from build123d import *

# Parameters (mm, degrees)
CROQUIS1_W              = 44.6
CROQUIS1_H              = 20.647373716
SALIENTE_EXTRUIR2_DEPTH = 10.5
CROQUIS2_R              = 7.366343287
CROQUIS2_R_2            = 3.5
SALIENTE_EXTRUIR3_DEPTH = 2
SALIENTE_EXTRUIR4_START = -2
CROQUIS3_R              = 6.292932571
CROQUIS3_R_2            = 3.5
SALIENTE_EXTRUIR4_DEPTH = 2
CORTAR_EXTRUIR1_DEPTH   = 5.5
CORTAR_EXTRUIR2_DEPTH   = 5.5
CROQUIS6_W              = 8
CROQUIS6_H              = 20.647373716
SALIENTE_EXTRUIR5_DEPTH = 3
CROQUIS7_W              = 8
CROQUIS7_H              = 20.647373716
SALIENTE_EXTRUIR6_DEPTH = 3
REDONDEO1_R             = 10
REDONDEO2_R             = 2


with BuildPart() as part:
    # Croquis1 → Saliente-Extruir2 (new body)
    with BuildSketch(Plane.XY):
        Rectangle(CROQUIS1_W, CROQUIS1_H)
        Polygon((5.946707773, 0), (2.973353886, 5.15), (-2.973353886, 5.15), (-5.946707773, 0), (-2.973353886, -5.15), (2.973353886, -5.15), align=None, mode=Mode.SUBTRACT)
    extrude(amount=SALIENTE_EXTRUIR2_DEPTH)

    # Croquis2 → Saliente-Extruir3 (add)
    with BuildSketch(Plane.XY.offset(10.5)):
        Circle(CROQUIS2_R)
        Circle(CROQUIS2_R_2, mode=Mode.SUBTRACT)
    extrude(amount=-SALIENTE_EXTRUIR3_DEPTH)

    # Croquis3 → Saliente-Extruir4 (add)
    with BuildSketch(Plane(origin=(0, 0, 0), x_dir=(-1, 0, 0), z_dir=(0, 0, -1)).offset(SALIENTE_EXTRUIR4_START)):
        Circle(CROQUIS3_R)
        with Locations(Location((0, 0, 0), (0, 0, 180))):
            Circle(CROQUIS3_R_2, mode=Mode.SUBTRACT)
    extrude(amount=SALIENTE_EXTRUIR4_DEPTH)

    # Croquis4 → Cortar-Extruir1 (cut)
    with BuildSketch(Plane(origin=(22.3, 0, 0), x_dir=(0, 0, -1), z_dir=(1, 0, 0))):
        Polygon((-5.25, 6.062177826), (-10.5, 3.031088913), (-10.5, -3.031088913), (-5.25, -6.062177826), (0, -3.031088913), (0, 3.031088913), align=None)
    extrude(amount=-CORTAR_EXTRUIR1_DEPTH, mode=Mode.SUBTRACT)

    # Croquis5 → Cortar-Extruir2 (cut)
    with BuildSketch(Plane.ZY.offset(22.3)):
        Polygon((5.25, 6.062177826), (0, 3.031088913), (0, -3.031088913), (5.25, -6.062177826), (10.5, -3.031088913), (10.5, 3.031088913), align=None)
    extrude(amount=-CORTAR_EXTRUIR2_DEPTH, mode=Mode.SUBTRACT)

    # Croquis6 → Saliente-Extruir5 (add)
    with BuildSketch(Plane(origin=(0, 0, 0), x_dir=(-1, 0, 0), z_dir=(0, 0, -1))):
        with Locations((-18.3, 0)):
            Rectangle(CROQUIS6_W, CROQUIS6_H)
        with Locations((18.3, 0)):
            Rectangle(CROQUIS6_W, CROQUIS6_H)
    extrude(amount=SALIENTE_EXTRUIR5_DEPTH)

    # Croquis7 → Saliente-Extruir6 (add)
    with BuildSketch(Plane.XY.offset(10.5)):
        with Locations((-18.3, 0)):
            Rectangle(CROQUIS7_W, CROQUIS7_H)
        with Locations((18.3, 0)):
            Rectangle(CROQUIS7_W, CROQUIS7_H)
    extrude(amount=SALIENTE_EXTRUIR6_DEPTH)

    # Redondeo1
    # the kernel refuses this fillet: 10 mm, written as the material it adds along each edge
    with BuildSketch(Plane(origin=(-14.3, 10.323686858, 10.5), x_dir=(1, 0, 0), z_dir=(0, -1, 0)), Plane(origin=(14.3, 10.323686858, 0), x_dir=(-1, 0, 0), z_dir=(0, -1, 0))) as redondeo1_piece_1:
        with BuildLine():
            CenterArc((7.141428429, 10), REDONDEO1_R, 224.427004001, 45.572995999)
            Line((0, 3), (-0.142828569, 2.86))
            ThreePointArc((-0.142828569, 2.86), (-0.2, 1.5), (-0.2, 0))
            Line((-0.2, 0), (0, -0.2))
            Line((0, -0.2), (7.141428429, -0.2))
            Line((7.141428429, -0.2), (7.141428429, 0))
        make_face()
    extrude(amount=20.647373716)
    with BuildSketch(Plane(origin=(14.3, 10.323686858, 10.5), x_dir=(0, 0, 1), z_dir=(0, -1, 0)), Plane(origin=(-14.3, 10.323686858, 0), x_dir=(0, 0, -1), z_dir=(0, -1, 0))) as redondeo1_piece_2:
        with BuildLine():
            CenterArc((10, 7.141428429), REDONDEO1_R, 180, 45.572995999)
            Line((0, 7.141428429), (-0.2, 7.141428429))
            Line((-0.2, 7.141428429), (-0.2, 0))
            Line((-0.2, 0), (0, -0.2))
            ThreePointArc((0, -0.2), (1.5, -0.2), (2.86, -0.142828569))
            Line((2.86, -0.142828569), (3, 0))
        make_face()
    extrude(amount=20.647373716)

    # Redondeo2
    redondeo2_edges = [part.edges().sort_by_distance(p)[0] for p in [
        (18.3, -10.323686858, -3),
        (18.3, 10.323686858, -3),
        (-18.3, 10.323686858, -3),
        (-18.3, -10.323686858, 13.5),
        (-18.3, 10.323686858, 13.5),
        (18.3, 10.323686858, 13.5),
        (18.3, -10.323686858, 13.5),
    ]]
    fillet(redondeo2_edges, radius=REDONDEO2_R)


solid = part.part
Can you work these out from the model? Positions are in its coordinate system, mm. A direction names the side the tool comes from. Coordinates: 2 decimals unless noted, no trailing zeros. Write each loop counter-clockwise with the first axis right and the second up, starting at its lowest first coordinate (ties: lowest second). Pieces come first, ordered by that corner, then holes. Notation, with made-up numbers: (20, 68) -> (69, 68) arc R10 cw to (69, 87) -> close; hole circle Ø3 at (43.5, 81). An arc over 180 degrees is marked (long way). Answer as CSV lines item,"result".
1) Will these pins go through, and if not, where does the flat tip stop? P1, Ø3, axis at y = 3, z = 6, coming from the -X side; P2, Ø9, axis at x = 0, y = 0, coming from the +Z side; P3, Ø5, axis at x = -14, y = 0, coming from the -Z side; P4, Ø3, axis at x = 6.5, y = -6.5, coming from the -Z side.
Check result:
P1,"x = -16.8"
P2,"z = 10.5"
P3,"z = -3"
P4,"z = -0.04"
2) On a 3-axis mill with a long thin cutter (end or side, diameter ignored), from which of +Z, -Z, +X, -X, +Y, -Y can I reach the whole of each face in a straight line? I mean faces 1 (the flat face through (-19.588, 4.525, 7.912)), 2 (the flat face through (0, 5.15, 5)), 3 (the flat face through (20, 0, 10.5)). Say none if no direction works.
Check result:
face 1,"-X"
face 2,"none"
face 3,"+X"
3) If I drill on line 1 (Y direction, x = 0, z = 1.6); line 2 (Y direction, x = 1, z = 7); line 3 (Z direction, x = 2.5, y = -6.5), over which ranges is the centre line in solid material (lowest first)? Write a range as from..to.
Check result:
line 1,"-10.32..-3.5, 3.5..10.32"
line 2,"-10.32..-5.15, 5.15..10.32"
line 3,"0..10.5"
4) If we section it at B-B on z = 9.25: Please give me the cut outline in (x, y).
Check result:
outline,"(-22.3, -10.32) -> (22.3, -10.32) -> (22.3, -3.75) -> (16.8, -3.75) -> (16.8, 3.75) -> (22.3, 3.75) -> (22.3, 10.32) -> (-22.3, 10.32) -> (-22.3, 3.75) -> (-16.8, 3.75) -> (-16.8, -3.75) -> (-22.3, -3.75) -> close; hole circle Ø7 at (0, 0)"
5) If we section it at D-D on z = 12: Please give me the cut outline in (x, y), then the cut area to 3 significant figures.
Check result:
outline,"(-22.3, -10.26) -> (-12.43, -10.26) -> (-12.43, 10.26) -> (-22.3, 10.26) -> close; (12.43, -10.26) -> (22.3, -10.26) -> (22.3, 10.26) -> (12.43, 10.26) -> close"
area,"405 mm²"
6) If we mould it in two halves opening along X, with no side actions, what happens to faces 4 (the flat face through (-19.588, -4.525, 2.588)), 5 (the flat face through (16.8, 0, 5)), 6 (the flat face through (0, 4, 8.5))? For each: +X half, -X half, draft (parallel to the pull), parting line (faces both ways), or undercut.
Check result:
face 4,"draft"
face 5,"+X half"
face 6,"undercut"
7) If we section it at A-A on x = 0: Please give me the cut outline in (y, z), then the cut area to 3 significant figures.
Check result:
outline,"(-10.32, 0) -> (-3.5, 0) -> (-3.5, 2) -> (-5.15, 2) -> (-5.15, 8.5) -> (-3.5, 8.5) -> (-3.5, 10.5) -> (-10.32, 10.5) -> close; (3.5, 0) -> (10.32, 0) -> (10.32, 10.5) -> (3.5, 10.5) -> (3.5, 8.5) -> (5.15, 8.5) -> (5.15, 2) -> (3.5, 2) -> close"
area,"122 mm²"
